For this review, take the finished solid that the model builds, in its own axes (mm). A direction names the side the tool comes from. Coordinates: 2 decimals unless noted, no trailing zeros. Loops run counter-clockwise (first coordinate to the right, second up) from the corner with the lowest first, then second, coordinate; pieces in that order, holes last. Notation, with made-up numbers: (53, -20) -> (95, -20) arc R13 ccw to (95, -3) -> close; hole circle Ø10 at (-7.75, -31.5). An arc over 180 degrees is marked (long way). Answer in a Markdown table with one row per item.
from build123d import *

# Parameters (mm, degrees)
SKETCH_1_W          = 5
SKETCH_1_H          = 10
SKETCH_1_W_2        = 10
SKETCH_1_H_2        = 5
EXTRUDE_1_DEPTH     = 5
SKETCH_1_3_W        = 5
SKETCH_1_3_H        = 10
SKETCH_1_3_W_2      = 10
SKETCH_1_3_H_2      = 5
EXTRUDE_2_DEPTH     = 20
CUT_EXTRUDE_1_DEPTH = 20
SCALE_1_SCALE       = 0.2


with BuildPart() as part:
    # Sketch 1 → Extrude 1 (new body)
    with BuildSketch(Plane(origin=(0, 0, 0), x_dir=(1, 0, 0), z_dir=(0, 1, 0))):
        with Locations((-15, 5)):
            Rectangle(SKETCH_1_W, SKETCH_1_H)
        Polygon((-12.5, 0), (2.5, 0), (7.5, 5), (7.5, 10), (-12.5, 10), align=None)
        Polygon((7.5, 5), (2.5, 0), (-12.5, 0), (-17.5, 0), (-17.5, -10), (17.5, -10), (17.5, 5), align=None)
        with Locations((12.5, 7.5)):
            Rectangle(SKETCH_1_W_2, SKETCH_1_H_2)
    extrude(amount=EXTRUDE_1_DEPTH)

    # Sketch 1_3 → Extrude 2 (add)
    with BuildSketch(Plane(origin=(0, 0, 0), x_dir=(1, 0, 0), z_dir=(0, 1, 0))):
        with Locations((-15, 5)):
            Rectangle(SKETCH_1_3_W, SKETCH_1_3_H)
        Polygon((-12.5, 0), (2.5, 0), (7.5, 5), (7.5, 10), (-12.5, 10), align=None)
        with Locations((12.5, 7.5)):
            Rectangle(SKETCH_1_3_W_2, SKETCH_1_3_H_2)
    extrude(amount=EXTRUDE_2_DEPTH)

    # Sketch 2 → Cut-Extrude 1 (cut)
    with BuildSketch(Plane.XY):
        with BuildLine():
            Line((-12.5, 20), (-2.5, 20))
            ThreePointArc((-2.5, 20), (-7.5, 15), (-12.5, 20))
        make_face()
        Polygon((17.5, 5), (7.5, 20), (17.5, 20), align=None)
    extrude(amount=-CUT_EXTRUDE_1_DEPTH, mode=Mode.SUBTRACT)


with BuildPart() as part_1:
    # Scale 1: scaled about (-1.822053886, 7.09893754, -2.737693345)
    add(part.part.scale(SCALE_1_SCALE).moved(Location((-1.457643109, 5.679150032, -2.190154676))))


solid = part_1.part
Item 1: Take a section at C-C, the plane x = -1.75. State the section outline as (y, z) points.
Worked answers:
| item | result |
|---|---|
| outline | (5.68, -4.19) -> (9.68, -4.19) -> (9.68, -2.19) -> (6.68, -2.19) -> (6.68, -0.19) -> (5.68, -0.19) -> close |
Item 2: Take a section at A-A, the plane y = 9.25. State the section outline as (x, z) points.
Worked answers:
| item | result |
|---|---|
| outline | (-4.96, -4.19) -> (-3.86, -4.19) -> (-3.86, -2.19) -> (-4.96, -2.19) -> close; (-2.05, -4.19) -> (0.33, -4.19) -> (0.33, -3.19) -> (0.04, -3.19) -> (-0.96, -2.19) -> (-2.05, -2.19) -> close |
Item 3: Insertion check: pin 1 (1.5 mm diameter, centred on x = -2.5, y = 9, fed in from +Z); pin 2 (2 mm diameter, centred on y = 8.5, z = -3.5, fed in from +X); pin 3 (0.9 mm diameter, centred on x = -2.5, z = -1, fed in from +Y); pin 4 (2 mm diameter, centred on x = 1.5, y = 7.5, fed in from +Z). Each pin has a flat end and moves straight along its axis. Give the tip position at first contact, or say it passes through.
Worked answers:
| item | result |
|---|---|
| pin 1 | z = -2.19 |
| pin 2 | x = 1.5 |
| pin 3 | y = 6.68 |
| pin 4 | z = -0.19 |
Item 4: For L1, parallel to Z at x = -4.25, y = 9; L2, parallel to Y at x = -1, z = -2; L3, parallel to X at y = 9.4, z = -2.9, list the stretches that pass through material, from the lowest coordinate up.
Worked answers:
| item | result |
|---|---|
| L1 | -4.19 to -2.19 |
| L2 | 5.68 to 6.68 |
| L3 | -4.96 to -3.92, -2 to -0.25 |
Item 5: For faces 1 (the flat face through (-4.5, 9.679, -3.2)), 2 (the flat face through (-3, 8, -2.19)), 3 (the flat face through (-2, 6.679, -1)), list the 3-axis set-ups (+Z, -Z, +X, -X, +Y, -Y) from which the entire face can be reached by the end or side of a thin tool; tool diameter is ignored.
Worked answers:
| item | result |
|---|---|
| face 1 | +Z, -Z, +X, -X, +Y |
| face 2 | +Z, +X, -X, +Y |
| face 3 | +Z, +X, +Y |
Item 6: Take a section at D-D, the plane y = 8.25. State the section outline as (x, z) points.
Worked answers:
| item | result |
|---|---|
| outline | (-4.96, -4.19) -> (1, -4.19) -> (1, -3.19) -> (0.04, -3.19) -> (-0.96, -2.19) -> (-4.96, -2.19) -> close |
Item 7: Take a section at B-B, the plane z = -3.5. State the section outline as (x, y) points.
Worked answers:
| item | result |
|---|---|
| outline | (-4.96, 5.68) -> (2.04, 5.68) -> (2.04, 6.68) -> (0.04, 9.68) -> (-1.96, 9.68) arc R1 cw to (-3.96, 9.68) -> (-4.96, 9.68) -> close |
Item 8: The part is to be moulded in two halves that separate along X. For faces 4 (the flat face through (-4.958, 7, -3)), 5 (the flat face through (0.8, 7.8, -3.19)), 6 (the cylindrical face through (-2.94, 8.68, -3.18)), say which applies: +X half, -X half, draft (parallel to the pull), parting line (faces both ways), or undercut.
Worked answers:
| item | result |
|---|---|
| face 4 | -X half |
| face 5 | draft |
| face 6 | undercut |
